Model file for the job. Use its own axes, mm. Face numbers are marked on the shaded views. A direction names the side the tool comes from. Round coordinates to 2 decimals unless told otherwise and drop trailing zeros. Loops run counter-clockwise (first coordinate to the right, second up) from the corner with the lowest first, then second, coordinate; pieces in that order, holes last. Notation, with made-up numbers: M -20.5,-1.75 L 33.5,-1.75 A10 ccw 33.5,17.25 Z; hole C 84,52 d2. An arc over 180 degrees is marked long. Answer in a Markdown table with one row per item.
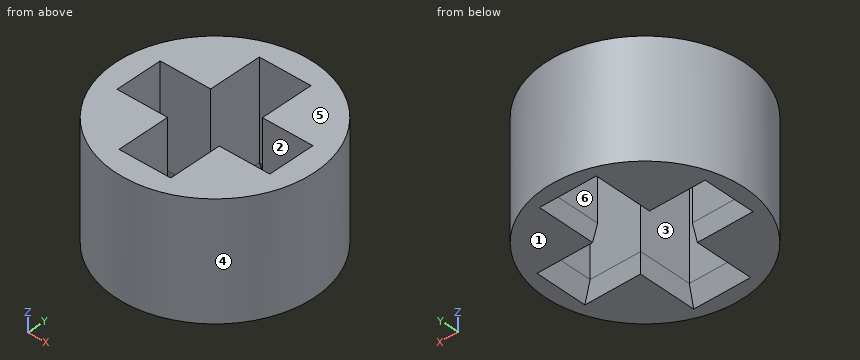
Autodesk Fusion 360 part; units mm, degrees
sketch "Sketch1" plane through (0, 0, 0) normal (0, 0, 1) x (1, 0, 0)
  line L0 (-0.715, 2.115) -> (0.715, 2.115)
  line L1 (0.715, 2.115) -> (0.715, -2.115)
  line L2 (0.715, -2.115) -> (-0.715, -2.115)
  line L3 (-0.715, -2.115) -> (-0.715, 2.115)
  line L4 (-0.715, 2.115) -> (0.715, -2.115) construction
  line L5 (0.715, 2.115) -> (-0.715, -2.115) construction
  line L6 (-2.115, 0.65) -> (2.115, 0.65)
  line L7 (2.115, 0.65) -> (2.115, -0.65)
  line L8 (2.115, -0.65) -> (-2.115, -0.65)
  line L9 (-2.115, -0.65) -> (-2.115, 0.65)
  line L10 (-2.115, 0.65) -> (2.115, -0.65) construction
  line L11 (2.115, 0.65) -> (-2.115, -0.65) construction
  circle A0 centre (0, 0) radius 2.75
  dimension "d21" = 1.43
  dimension "d22" = 4.23
  dimension "d23" = 4.23
  dimension "d24" = 1.3
  dimension "d25" = 5.5
extrude "Extrude1" add sketch "Sketch1" against normal blind 3.2
chamfer "Chamfer1" distance 0.212 angle 67.02 4 edges at (-2.115, 0, -3.2) (2.115, 0, -3.2) (0, -2.115, -3.2) (0, 2.115, -3.2) measured on face at (-1.6153, -1.0568, -3.2) measured on face at (-1.6153, -1.0568, -3.2) measured on face at (-1.6153, -1.0568, -3.2) measured on face at (-1.6153, -1.0568, -3.2)
chamfer "Chamfer2" distance 0.072 angle 81.8 8 edges at (0.715, 1.4885, -3.2) (1.521, 0.65, -3.2) (1.521, -0.65, -3.2) (0.715, -1.4885, -3.2) (-0.715, -1.4885, -3.2) (-1.521, -0.65, -3.2) (-1.521, 0.65, -3.2) (-0.715, 1.4885, -3.2) measured on face at (-1.0482, 1.709, -3.2) measured on face at (-1.0482, 1.709, -3.2) measured on face at (-1.0482, 1.709, -3.2) measured on face at (-1.0482, 1.709, -3.2) measured on face at (-1.0482, 1.709, -3.2) measured on face at (-1.0482, 1.709, -3.2) measured on face at (-1.0482, 1.709, -3.2) measured on face at (-1.0482, 1.709, -3.2)
equation "width = 5.5 mm"
equation "depth = 5.5 mm"
equation "cross_xy = 4.23 mm"
equation "gap_x = 1.3 mm"
equation "gap_y = 1.43 mm"
equation "height = 3.2 mm"
equation "d15 = chamfer_cross"
equation "d16 = chamfer_cross_angle"
equation "d17 = chamfer_gap"
equation "d18 = chamfer_gap_angle"
equation "d21 = gap_y"
equation "d22 = cross_xy"
equation "d23 = cross_xy"
equation "d24 = gap_x"
equation "d25 = width"
equation "chamfer_cross_angle = 67.02 deg"
equation "chamfer_cross = 0.212 mm"
equation "chamfer_gap_angle = 81.8 deg"
equation "chamfer_gap = 0.072 mm"
1. Wall check: probe 1 along Y at (x, z) = (0.1, -2.45) (3 decimals); probe 2 along X at (y, z) = (-1.7, -2.4) (3 decimals); probe 3 along X at (y, z) = (0.5, -2.15) (3 decimals). Give the ranges that are in metal, low to high.
Verdict:
| item | result |
|---|---|
| probe 1 | y = -2.748 to -2.115, 2.115 to 2.748 |
| probe 2 | x = -2.162 to -0.715, 0.715 to 2.162 |
| probe 3 | x = -2.704 to -2.115, 2.115 to 2.704 |
2. Saw through at C-C (x = -1.65). Write the cut outline in (y, z).
Verdict:
| item | result |
|---|---|
| outline | M -2.2,-3.2 L -0.72,-3.2 L -0.65,-2.7 L -0.65,0 L -2.2,0 Z; M 0.65,-2.7 L 0.72,-3.2 L 2.2,-3.2 L 2.2,0 L 0.65,0 Z |
3. Mould opens along X. For the marked faces 3, 4, 5 and 6 say: +X half, -X half, draft (parallel to the pull), parting line (faces both ways), or undercut.
Verdict:
| item | result |
|---|---|
| face 3 | undercut |
| face 4 | parting line |
| face 5 | draft |
| face 6 | undercut |
4. Saw through at A-A (y = 0). Write the cut outline in (x, z) (3 decimals), and give its area (3 significant figures).
Verdict:
| item | result |
|---|---|
| outline | M -2.75,-3.2 L -2.327,-3.2 L -2.115,-2.7 L -2.115,0 L -2.75,0 Z; M 2.115,-2.7 L 2.327,-3.2 L 2.75,-3.2 L 2.75,0 L 2.115,0 Z |
| area | 3.96 mm² |
5. Tool access for the marked faces 1 and 2: list every direction of +Z, -Z, +X, -X, +Y, -Y with a clear straight run to the whole face (end or side of a thin tool).
Verdict:
| item | result |
|---|---|
| face 1 | -Z, +X, -X, +Y, -Y |
| face 2 | +Z, -Z |
6. Saw through at B-B (z = -1.3). Write the cut outline in (x, y) (3 decimals).
Verdict:
| item | result |
|---|---|
| outline | C 0,0 d5.5; hole M -2.115,-0.65 L -0.715,-0.65 L -0.715,-2.115 L 0.715,-2.115 L 0.715,-0.65 L 2.115,-0.65 L 2.115,0.65 L 0.715,0.65 L 0.715,2.115 L -0.715,2.115 L -0.715,0.65 L -2.115,0.65 Z |
7. Saw through at D-D (x = 2.4). Write the cut outline in (y, z), and give its area (3 significant figures).
Verdict:
| item | result |
|---|---|
| outline | M -1.34,-3.2 L 1.34,-3.2 L 1.34,0 L -1.34,0 Z |
| area | 8.59 mm² |
8. Pin check, flat tips, straight feed: pin 1 (1.1 mm diameter, centred on x = -1.5, z = -1.5, fed in from +Y); pin 2 (1.6 mm diameter, centred on y = 1, z = -2, fed in from +X); pin 3 (0.7 mm diameter, centred on x = -1.5, z = -1, fed in from -Y). Stop position of each tip, or through.
Verdict:
| item | result |
|---|---|
| pin 1 | stops at y = 2.58 |
| pin 2 | stops at x = 2.74 |
| pin 3 | stops at y = -2.5 |
